Design review of the part built by this model. Coordinates are the model's own, in mm. A direction names the side the tool comes from. Give positions to 0.01 mm unless a question says otherwise; leave off trailing zeros. Loops run counter-clockwise (first coordinate to the right, second up) from the corner with the lowest first, then second, coordinate; pieces in that order, holes last.
from build123d import *

# Parameters (mm, degrees)
F0_R     = 20
F0_R_2   = 15
F1_DEPTH = 5
F2_R     = 4.99999
F3_START = 40
F3_DEPTH = 25
F0_R_3   = 12.5
F4_DEPTH = 65
F5_R     = 3


# Not quite as in the source:
# - a fillet or chamfer that OpenCascade refuses, or shapes differently, is made with other operations: its cross-section is extruded or revolved along the edge and cut away or added
# - a fillet or chamfer is up to 0.001 mm smaller than in the source, because OpenCascade refuses the exact size


with BuildPart() as f1:
    # F0 (on Top) → F1 (new body)
    with BuildSketch(Plane.XY):
        with BuildLine():
            add(Edge.make_bspline(
                [(-22.8928557761, -15.2370323363), (-16.7035213729, -41.1210767925), (0, -41.1210767925)],
                knots=[5.091980066, 5.091980066, 5.091980066, 6.2831853072, 6.2831853072, 6.2831853072], degree=2, weights=[1, 0.8278105744, 1]))
            add(Edge.make_bspline(
                [(0, -41.1210767925), (16.7035213729, -41.1210767925), (22.8928557761, -15.2370323363)],
                knots=[0, 0, 0, 1.1912052412, 1.1912052412, 1.1912052412], degree=2, weights=[1, 0.8278105744, 1]))
            ThreePointArc((22.8928557761, -15.2370323363), (0, -27.5), (-22.8928557761, -15.2370323363))
        make_face()
        with BuildLine():
            ThreePointArc((-22.8928557761, 15.2370323363), (0, 27.5), (22.8928557761, 15.2370323363))
            add(Edge.make_bspline(
                [(22.8928557761, 15.2370323363), (0, 110.9758724176), (-22.8928557761, 15.2370323363)],
                knots=[1.9503874124, 1.9503874124, 1.9503874124, 4.3327978948, 4.3327978948, 4.3327978948], degree=2, weights=[1, 0.3705406941, 1]))
        make_face()
        with BuildLine():
            ThreePointArc((-22.8928557761, -15.2370323363), (0, -27.5), (22.8928557761, -15.2370323363))
            add(Edge.make_bspline(
                [(22.8928557761, -15.2370323363), (26.5363006249, 0), (22.8928557761, 15.2370323363)],
                knots=[1.1912052412, 1.1912052412, 1.1912052412, 1.9503874124, 1.9503874124, 1.9503874124], degree=2, weights=[1, 0.9288162326, 1]))
            ThreePointArc((22.8928557761, 15.2370323363), (0, 27.5), (-22.8928557761, 15.2370323363))
            add(Edge.make_bspline(
                [(-22.8928557761, 15.2370323363), (-26.5363006249, 0), (-22.8928557761, -15.2370323363)],
                knots=[4.3327978948, 4.3327978948, 4.3327978948, 5.091980066, 5.091980066, 5.091980066], degree=2, weights=[1, 0.9288162326, 1]))
        make_face()
        Circle(F0_R, mode=Mode.SUBTRACT)
        Circle(F0_R)
        Circle(F0_R_2, mode=Mode.SUBTRACT)
    extrude(amount=F1_DEPTH)

    # F2 (radius 5 in the source; OpenCascade refuses exactly that, so slightly less here)
    f2_edges = [f1.edges().sort_by_distance(p)[0] for p in [
        (-22.892856, 15.237032, 5),
    ]]
    fillet(f2_edges, radius=F2_R)



with BuildPart() as f3:
    # F0 (on Top) → F3 (new body)
    with BuildSketch(Plane.XY.offset(F3_START)):
        Circle(F0_R)
        Circle(F0_R_2, mode=Mode.SUBTRACT)
    extrude(amount=F3_DEPTH)


with BuildPart() as f1_1:
    add(f1.part)

    add(f3.part)  # F4 merges F3
    # F0 (on Top) → F4 (join)
    with BuildSketch(Plane.XY):
        Circle(F0_R_2)
        Circle(F0_R_3, mode=Mode.SUBTRACT)
    extrude(amount=F4_DEPTH)

    # F5
    f5_edges = [f1_1.edges().sort_by_distance(p)[0] for p in [
        (-12.5, 0, 65),
    ]]
    fillet(f5_edges, radius=F5_R)

    # F6: fillet of radius 17 on 3 edges, made by hand

    # F6_s1 → F6_t2 (revolve, cut)
    with BuildSketch(Plane.XZ):
        with BuildLine():
            ThreePointArc((20, 52.0415945788), (18.7003184681, 45.5223921736), (15, 40))
            Line((15, 40), (15.24, 39.7591681084))
            ThreePointArc((15.24, 39.7591681084), (17.5, 39.66), (20, 39.66))
            Line((20, 39.66), (20.34, 40))
            Line((20.34, 40), (20.34, 52.0415945788))
            Line((20.34, 52.0415945788), (20, 52.0415945788))
        make_face()
    revolve(axis=Axis((0, 0, 40), (0, 0, 1)), mode=Mode.SUBTRACT)

    # F6_s3 → F6_t4 (revolve, cut)
    with BuildSketch(Plane.XZ):
        with BuildLine():
            ThreePointArc((15.5, 65), (18.8350876221, 59.6629398166), (20, 53.4782813782))
            Line((20, 53.4782813782), (20.34, 53.4782813782))
            Line((20.34, 53.4782813782), (20.34, 65))
            Line((20.34, 65), (20, 65.34))
            ThreePointArc((20, 65.34), (17.75, 65.34), (15.75, 65.2304343724))
            Line((15.75, 65.2304343724), (15.5, 65))
        make_face()
    revolve(axis=Axis((0, 0, 65), (0, 0, 1)), mode=Mode.SUBTRACT)


solid = f1_1.part
Q1. Insertion check: pin 1 (6 mm diameter, centred on x = -14, z = 38, fed in from +Y); pin 2 (1.5 mm diameter, centred on x = -1, y = -11, fed in from -Z); pin 3 (6 mm diameter, centred on x = 8.5, y = -5.5, fed in from -Z); pin 4 (5 mm diameter, centred on x = -9, y = -27.5, fed in from +Z). Each pin has a flat end and moves straight along its axis. Give the tip position at first contact, or say it passes through.
Results:
pin 1: stops at y = 10.2
pin 2: passes through
pin 3: stops at z = 0
pin 4: stops at z = 5
Q2. Take a section at A-A (z = 6). Give the boundary of the cut face in (x, y), plus the area to 3 significant figures.
Results:
outline: circle Ø30 at (0, 0); hole circle Ø25 at (0, 0)
area: 216 mm2
Q3. Wall thickness on line 1 (X direction, y = 0.5, z = 20); line 2 (Y direction, x = 0, z = 32); line 3 (X direction, y = -23.5, z = 4): over which ranges is each line inside the solid? List them lowest first.
Results:
line 1: x = -14.99 to -12.49, 12.49 to 14.99
line 2: y = -15 to -12.5, 12.5 to 15
line 3: x = -18.05 to 18.05
Q4. Tool access review of faces 1 (the face through (-4.336, -19.524, 52.75)), 2 (the face through (0, 13, 0)): name each direction out of +Z, -Z, +X, -X, +Y, -Y from which nothing blocks a thin tool from reaching the whole face with its end or side.
Results:
face 1: +Z
face 2: -Z, +X, -X, +Y, -Y
Q5. Draft analysis for pull direction X (two halves, no side actions). For faces 3 (the face through (11.923, 3.755, 30.566)), 4 (the face through (0, -16, 5)), 5 (the face through (-14.985, 0.66, 22.255)), state which applies: pulls with the +X half, pulls with the -X half, needs draft (parallel to the pull), parting line crosses it, or undercut.
Results:
face 3: undercut
face 4: needs draft
face 5: parting line crosses it
